Source: CAD feature listing. Evaluate the final solid. Frame: model axes, mm. A direction names the side the tool comes from. Give positions to 0.01 mm unless a question says otherwise; leave off trailing zeros. Order: outer loops, then holes, each group sorted by start corner. A loop starts at its lowest first (then second) coordinate and runs counter-clockwise, first axis right, second up. Notation, with made-up numbers: M 81.25,6.5 L 133.25,6.5 A27 cw 133.25,24.5 Z; hole C 40.5,4.25 d11. An arc over 180 degrees is marked long. Return JSON: item names as keys, results as strings.
Autodesk Fusion 360 part; units mm, degrees
sketch "スケッチ1" plane through (0, 0, 0) normal (0, 0, 1) x (1, 0, 0)
  line L0 (-38.8909, 38.8909) -> (0, 0)
  line L1 (0, 0) -> (38.8909, 38.8909)
  line L2 (38.8909, 38.8909) -> (-38.8909, 38.8909) construction
  line L3 (0, 38.8909) -> (0, 0) construction
  line L4 (-24.5921, 31.6632) -> (-3.3789, 10.45)
  line L5 (-3.3789, 10.45) -> (3.3789, 10.45)
  line L6 (3.3789, 10.45) -> (24.5921, 31.6632)
  line L7 (24.5921, 31.6632) -> (24.5921, 38.8909)
  line L8 (-24.5921, 38.8909) -> (-24.5921, 31.6632)
  line L9 (-24.5921, 38.8909) -> (24.5921, 38.8909)
  line L10 (-38.8909, 38.8909) -> (-38.8909, 45.9909)
  line L11 (-31.8909, 45.9909) -> (31.8909, 45.9909)
  line L12 (38.8909, 45.9909) -> (38.8909, 38.8909)
  line L13 (31.8909, 45.9909) -> (-31.8909, 45.9909)
  line L14 (-38.8909, 45.9909) -> (-38.8909, 95.9909)
  line L15 (-38.8909, 95.9909) -> (38.8909, 95.9909)
  line L16 (38.8909, 95.9909) -> (38.8909, 45.9909)
  line L17 (38.8909, 45.9909) -> (-38.8909, 95.9909) construction
  line L18 (-38.8909, 45.9909) -> (38.8909, 95.9909) construction
  line L19 (-31.8909, 45.9909) -> (-31.8909, 81.9198)
  line L20 (-24.8198, 88.9909) -> (24.8198, 88.9909)
  line L21 (31.8909, 81.9198) -> (31.8909, 45.9909)
  line L22 (-24.8198, 88.9909) -> (-31.8909, 81.9198)
  line L23 (24.8198, 88.9909) -> (31.8909, 81.9198)
  point P0 (0, 70.9909)
  point P1 (0, 70.9909)
  dimension "d1" = 55
  dimension "d3" = 55
  dimension "d4" = 5
  dimension "d5" = 5
  dimension "d6" = 30
  dimension "d7" = 30
  dimension "d8" = 10.45
  dimension "d9" = 7.1
  dimension "d10" = 50
  dimension "d11" = 7
  dimension "d13" = 45
  dimension "d14" = 45
  dimension "d15" = 10
  dimension "d16" = 10
  dimension "d17" = 7
  dimension "d18" = 7
  dimension "d19" = 57.1
  dimension "d20" = 7.1
extrude "押し出し1" add sketch "スケッチ1" along normal mid plane 5
sketch "スケッチ2" plane through (0, 0, 2.5) normal (0, 0, 1) x (1, 0, 0)
  line L0 (-31.8909, 81.9198) -> (-24.8198, 88.9909)
  line L1 (-24.8198, 88.9909) -> (24.8198, 88.9909)
  line L2 (24.8198, 88.9909) -> (31.8909, 81.9198)
  line L3 (31.8909, 81.9198) -> (31.8909, 45.9909)
  line L4 (31.8909, 45.9909) -> (-31.8909, 45.9909)
  line L5 (-31.8909, 45.9909) -> (-31.8909, 81.9198)
  line L6 (-3.3789, 10.45) -> (-24.5921, 31.6632)
  line L7 (-24.5921, 31.6632) -> (-24.5921, 38.8909)
  line L8 (-24.5921, 38.8909) -> (24.5921, 38.8909)
  line L9 (24.5921, 38.8909) -> (24.5921, 31.6632)
  line L10 (24.5921, 31.6632) -> (3.3789, 10.45)
  line L11 (3.3789, 10.45) -> (-3.3789, 10.45)
  line L12 (-38.8909, 38.8909) -> (0, 0)
  line L13 (0, 0) -> (38.8909, 38.8909)
  line L14 (38.8909, 38.8909) -> (38.8909, 95.9909)
  line L15 (38.8909, 95.9909) -> (-38.8909, 95.9909)
  line L16 (-38.8909, 95.9909) -> (-38.8909, 38.8909)
  line L17 (-24.8198, 95.9909) -> (-24.8198, 88.9909)
  line L18 (-24.8198, 88.9909) -> (-31.8909, 81.9198)
  line L19 (-31.8909, 81.9198) -> (-38.8909, 81.9198)
  line L20 (-38.8909, 81.9198) -> (-38.8909, 95.9909)
  line L21 (-38.8909, 95.9909) -> (-24.8198, 95.9909)
  line L22 (24.8198, 95.9909) -> (24.8198, 88.9909)
  line L23 (24.8198, 88.9909) -> (31.8909, 81.9198)
  line L24 (31.8909, 81.9198) -> (38.8909, 81.9198)
  line L25 (38.8909, 81.9198) -> (38.8909, 95.9909)
  line L26 (38.8909, 95.9909) -> (24.8198, 95.9909)
  line L27 (-24.5921, 45.9909) -> (-24.5921, 31.6632)
  line L28 (-24.5921, 31.6632) -> (-31.6632, 31.6632)
  line L29 (-31.6632, 31.6632) -> (-38.8909, 38.8909)
  line L30 (-38.8909, 38.8909) -> (-38.8909, 45.9909)
  line L31 (-38.8909, 45.9909) -> (-24.5921, 45.9909)
  line L32 (24.5921, 45.9909) -> (24.5921, 31.6632)
  line L33 (24.5921, 31.6632) -> (31.6632, 31.6632)
  line L34 (31.6632, 31.6632) -> (38.8909, 38.8909)
  line L35 (38.8909, 38.8909) -> (38.8909, 45.9909)
  line L36 (38.8909, 45.9909) -> (24.5921, 45.9909)
  line L37 (-3.3789, 10.45) -> (-6.9145, 6.9145)
  line L38 (-6.9145, 6.9145) -> (0, 0)
  line L39 (0, 0) -> (6.9145, 6.9145)
  line L40 (6.9145, 6.9145) -> (3.3789, 10.45)
  line L41 (3.3789, 10.45) -> (-3.3789, 10.45)
extrude "押し出し2" add sketch "スケッチ2" along normal blind 15 contours L0 L15 L16 L17 L18 L19 L20 L21 | L4 L7 L12 L16 L27 L28 L29 L30 L31 | L2 L14 L15 L22 L23 L24 L25 L26 | L4 L9 L13 L14 L32 L33 L34 L35 L36
extrude "押し出し3" add sketch "スケッチ2" along normal blind 60 contours L11 L12 L13 L37 L38 L39 L40 L41
sketch "スケッチ3" plane through (0, 0, -2.5) normal (0, 0, -1) x (-1, 0, 0)
  line L0 (24.8198, 88.9909) -> (31.8909, 81.9198)
  line L1 (31.8909, 81.9198) -> (31.8909, 45.9909)
  line L2 (31.8909, 45.9909) -> (-31.8909, 45.9909)
  line L3 (-31.8909, 45.9909) -> (-31.8909, 81.9198)
  line L4 (-31.8909, 81.9198) -> (-24.8198, 88.9909)
  line L5 (-24.8198, 88.9909) -> (24.8198, 88.9909)
  line L6 (24.5921, 31.6632) -> (3.3789, 10.45)
  line L7 (3.3789, 10.45) -> (-3.3789, 10.45)
  line L8 (-3.3789, 10.45) -> (-24.5921, 31.6632)
  line L9 (-24.5921, 31.6632) -> (-24.5921, 38.8909)
  line L10 (-24.5921, 38.8909) -> (24.5921, 38.8909)
  line L11 (24.5921, 38.8909) -> (24.5921, 31.6632)
  line L12 (0, 0) -> (38.8909, 38.8909)
  line L13 (38.8909, 38.8909) -> (38.8909, 95.9909)
  line L14 (38.8909, 95.9909) -> (-38.8909, 95.9909)
  line L15 (-38.8909, 95.9909) -> (-38.8909, 38.8909)
  line L16 (-38.8909, 38.8909) -> (0, 0)
  line L17 (-38.8909, 95.9909) -> (-28.3553, 85.4553) construction
  line L18 (38.8909, 95.9909) -> (28.3553, 85.4553) construction
  circle A0 centre (-33.6231, 90.7231) radius 3.5
  circle A1 centre (33.6231, 90.7231) radius 3.5
  circle A2 centre (-31.8909, 38.8909) radius 3.5
  circle A3 centre (31.8909, 38.8909) radius 3.5
  line L19 (-24.5921, 38.8909) -> (-38.8909, 38.8909) construction
  line L20 (-31.8909, 45.9909) -> (-31.8909, 31.8909) construction
  line L21 (24.5921, 38.8909) -> (38.8909, 38.8909) construction
  line L22 (31.8909, 45.9909) -> (31.8909, 31.8909) construction
  circle A4 centre (-31.8909, 38.8909) radius 1.5
  circle A5 centre (31.8909, 38.8909) radius 1.5
  circle A6 centre (33.6231, 90.7231) radius 1.5
  circle A7 centre (-33.6231, 90.7231) radius 1.5
  dimension "d27" = 7
  dimension "d28" = 7
  dimension "d29" = 7
  dimension "d30" = 7
  dimension "d31" = 3
  dimension "d32" = 3
  dimension "d33" = 3
  dimension "d34" = 3
extrude "押し出し4" cut sketch "スケッチ3" against normal blind 25 contours A4 | A5 | A6 | A7
extrude "押し出し7" cut 1 faces at (0, 6.9667, 62.5) along direction (0, 0, -1) blind 65
sketch "スケッチ8" plane through (0, 0, 2.5) normal (0, 0, 1) x (1, 0, 0)
  line L0 (-6.9145, 6.9145) -> (-3.3789, 10.45)
  line L1 (-3.3789, 10.45) -> (-24.5921, 31.6632)
  line L2 (-24.5921, 31.6632) -> (-31.6632, 31.6632)
  line L3 (-31.6632, 31.6632) -> (-6.9145, 6.9145)
  line L4 (3.3789, 10.45) -> (6.9145, 6.9145)
  line L5 (24.5921, 31.6632) -> (3.3789, 10.45)
  line L6 (6.9145, 6.9145) -> (31.6632, 31.6632)
  line L7 (-3.3789, 10.45) -> (3.3789, 10.45)
  line L8 (-6.9145, 13.9855) -> (6.9145, 13.9855)
  line L9 (6.9145, 13.9855) -> (10.45, 10.45)
  line L10 (-6.9145, 13.9855) -> (-10.45, 10.45)
  dimension "d52" = 5
  dimension "d53" = 5
extrude "押し出し9" add sketch "スケッチ8" against normal blind 5 contours L1 L5 L7 L8
extrude "押し出し10" add sketch "スケッチ8" along normal blind 20 contours L0 L1 L3 L10 | L1 L5 L7 L8 | L4 L5 L6 L9
sketch "スケッチ9" plane through (0, 10.45, 0) normal (0, -1, 0) x (1, 0, 0)
  line L0 (-3.3789, 22.5) -> (-3.3789, -2.5)
  line L1 (-3.3789, -2.5) -> (3.3789, -2.5)
  line L2 (3.3789, -2.5) -> (3.3789, 22.5)
  line L3 (3.3789, 22.5) -> (-3.3789, 22.5)
  arc A0 (-1.5, 7.5) -> (1.5, 7.5) centre (0, 7.5) ccw
  line L4 (0, 7.5) -> (0, -2.5) construction
  line L5 (-1.5, 7.5) -> (-1.5, 22.5)
  line L6 (1.5, 22.5) -> (1.5, 7.5)
  dimension "d58" = 10
  dimension "d59" = 1.5
extrude "押し出し11" cut sketch "スケッチ9" against normal blind 4 contours L3 A0 L5 L6
extrude "押し出し12" add sketch "スケッチ3" against normal blind 4 contours A4 | A5 | A6 | A7
1. First-contact query: pin 1 (3.5 mm diameter, centred on x = -34.5, y = 91, fed in from +Z); pin 2 (12 mm diameter, centred on x = 14, y = 29, fed in from +Z); pin 3 (2.5 mm diameter, centred on x = 11.5, z = 0.5, fed in from -Y). Flat tips, straight axial feed; report the tip coordinate or a pass-through.
Evaluation:
{"pin 1": "stops at z = 17.5", "pin 2": "stops at z = 2.5", "pin 3": "stops at y = 10.25"}
2. Ray query, probe 1 along X at (y, z) = (90.5, 5.5); probe 2 along X at (y, z) = (39, 14.25); probe 3 along Y at (x, z) = (-8, 2.25). Return the intervals inside material, ascending.
Evaluation:
{"probe 1": "x = -38.89 to -35.11, -32.14 to -24.82, 24.82 to 32.14, 35.11 to 38.89", "probe 2": "x = -38.89 to -33.39, -30.39 to -24.59, 24.59 to 30.39, 33.39 to 38.89", "probe 3": "y = 8 to 15.07, 38.89 to 45.99, 88.99 to 95.99"}
3. Set-up query: faces 4 (the face through (-32, 39, 1.5)), 5 (the face through (-28.31, 85.5, 7.36)), 6 (the face through (28, 31.663, 10)), 7 (the face through (1.5, 12, 15)). Return all of +Z, -Z, +X, -X, +Y, -Y with unobstructed straight access to the full face (end or side cutting, diameter ignored); none if empty.
Evaluation:
{"face 4": "+Z", "face 5": "+Z, -Z", "face 6": "+Z, +X, -X, -Y", "face 7": "+Z, +Y, -Y"}
4. Section query B-B (y = 62). Return loops of the section in (x, z).
Evaluation:
{"outline": "M -38.89,-2.5 L -31.89,-2.5 L -31.89,2.5 L -38.89,2.5 Z; M 31.89,-2.5 L 38.89,-2.5 L 38.89,2.5 L 31.89,2.5 Z"}
5. Section query C-C (y = 21). Return loops of the section in (x, z).
Evaluation:
{"outline": "M -21,-2.5 L -13.93,-2.5 L -13.93,2.5 L -21,2.5 Z; M 13.93,-2.5 L 21,-2.5 L 21,2.5 L 13.93,2.5 Z"}
6. Draft query along X for faces 1 (the face through (8.7, 12.2, 12.4)), 2 (the face through (32, 89, 17.5)), 3 (the face through (24.592, 39, 7)). Return one class per face: pulls with the +X half, pulls with the -X half, needs draft (parallel to the pull), parting line crosses it, or undercut.
Evaluation:
{"face 1": "pulls with the +X half", "face 2": "needs draft", "face 3": "undercut"}
7. Section query D-D (z = 15.75). State how many separate pieces and enclosed holes the cut face has, then the cut area to 3 significant figures.
Evaluation:
{"separate pieces": "6", "enclosed holes": "4", "area": "751 mm^2"}
8. Section query A-A (x = 0). Return loops of the section in (y, z).
Evaluation:
{"outline": "M 10.45,-2.5 L 13.99,-2.5 L 13.99,6 L 10.45,6 Z; M 38.89,-2.5 L 45.99,-2.5 L 45.99,2.5 L 38.89,2.5 Z; M 88.99,-2.5 L 95.99,-2.5 L 95.99,2.5 L 88.99,2.5 Z"}
